Design review of the part built by this model. Coordinates are the model's own, in mm. Face numbers are marked on the shaded views. A direction names the side the tool comes from. Coordinates: 2 decimals unless noted, no trailing zeros. Loops run counter-clockwise (first coordinate to the right, second up) from the corner with the lowest first, then second, coordinate; pieces in that order, holes last. Notation, with made-up numbers: (45, -0.5) -> (87, -0.5) arc R15 cw to (87, 5.5) -> close; hole circle Ø3 at (-14.5, -9). An arc over 180 degrees is marked (long way). Use one line per item in the form item = value. Start each with the question number.
1. Consider section D-D (x = 3.5). State the section outline as (y, z) points, then the cut area to 3 significant figures.
2. Wall thickness on line 1 (Y direction, x = -13.65, z = 73.05) (3 decimals); line 2 (Y direction, x = 19.4, z = 25.05); line 3 (Z direction, x = -13, y = -13): over which ranges is each line inside the solid? List them lowest first. Write a range as from..to.
3. Machinability: for the marked faces 1, 2 and 3, which of the approach directions +Z, -Z, +X, -X, +Y, -Y give a long, thin tool a straight path to every point of the face, cutting with its end or side? Answer none if there is none.
4. Consider section B-B (y = 29.95). State the section outline as (x, z) points (3 decimals).
5. Consider section A-A (x = 17.47). State the section outline as (y, z) points.
6. Consider section C-C (z = 53). State the section outline as (x, y) points (3 decimals).
7. For pin 1 (2 mm diameter, centred on y = 4, z = 44.5, fed in from -X); pin 2 (12 mm diameter, centred on x = 10, z = 56, fed in from +Y); pin 3 (1.6 mm diameter, centred on x = 12.5, y = 6, fed in from +Z); pin 4 (2 mm diameter, centred on y = 29.95, z = 73.05, fed in from -X), all flat-tipped, find the tip position at first contact; note any pin that passes through.
from build123d import *

# Parameters (mm, degrees)
SKETCH1_W           = 11
SKETCH1_H           = 17
SKETCH1_W_2         = 7
SKETCH1_H_2         = 13
BOSS_EXTRUDE1_DEPTH = 76.2
SKETCH2_W           = 11
SKETCH2_H           = 17
BOSS_EXTRUDE2_DEPTH = 2
SKETCH3_W           = 7
SKETCH3_H           = 11
CUT_EXTRUDE1_DEPTH  = 2
SKETCH4_W           = 38.1
SKETCH4_H           = 38.1
SKETCH4_W_2         = 11
SKETCH4_H_2         = 17
BOSS_EXTRUDE3_DEPTH = 3
SKETCH5_R           = 12.7
SKETCH5_W           = 11
SKETCH5_H           = 17
BOSS_EXTRUDE4_DEPTH = 2.54
SKETCH6_W           = 11
SKETCH6_H           = 58.214
BOSS_EXTRUDE5_DEPTH = 6.35
CUT_EXTRUDE2_REACH  = 87.303
SKETCH7_R           = 3.302
SKETCH8_W           = 6.985
SKETCH8_H           = 31.75
CUT_EXTRUDE3_DEPTH  = 6.35
SKETCH9_W           = 58.42
SKETCH9_H           = 12.7
BOSS_EXTRUDE6_DEPTH = 12.7
SKETCH10_W          = 3.175
SKETCH10_H          = 58.214
BOSS_EXTRUDE7_DEPTH = 20
SKETCH11_R          = 1.778
SKETCH11_W          = 3.884096392
SKETCH11_H          = 20
CUT_EXTRUDE4_DEPTH  = 91.512682122
FILLET1_R           = 1.27
CHAMFER1_SIZE       = 11.43
FILLET3_R           = 2.54
SKETCH12_W          = 58.214
SKETCH12_H          = 11.675
BOSS_EXTRUDE8_DEPTH = 12.7
SKETCH13_W          = 3.175
SKETCH13_H          = 54.356
BOSS_EXTRUDE9_DEPTH = 20
CHAMFER3_SIZE       = 12.7
FILLET4_R           = 2.54
SKETCH14_W          = 6.096
SKETCH14_H          = 28.594092226
CUT_EXTRUDE5_DEPTH  = 6.35
SKETCH15_R          = 1.778
CUT_EXTRUDE6_DEPTH  = 91.512682122
FILLET5_R           = 1.27
SKETCH16_R          = 1.5875
CUT_EXTRUDE7_DEPTH  = 12.7
FILLET6_R           = 2.54
SKETCH17_R          = 3.302
CUT_EXTRUDE8_DEPTH  = 72.570750283
SKETCH19_W          = 11
SKETCH19_H          = 17
CUT_EXTRUDE9_DEPTH  = 2.032
SKETCH21_W          = 41.629903608
SKETCH21_H          = 20
CUT_EXTRUDE10_DEPTH = 25.4
SKETCH22_W          = 41.656
SKETCH22_H          = 20
CUT_EXTRUDE11_DEPTH = 25.4


with BuildPart() as part:
    # Sketch1 → Boss-Extrude1 (new body)
    with BuildSketch(Plane.XY):
        with Locations((3.5, 6.5)):
            Rectangle(SKETCH1_W, SKETCH1_H)
        with Locations((3.5, 6.5)):
            Rectangle(SKETCH1_W_2, SKETCH1_H_2, mode=Mode.SUBTRACT)
    extrude(amount=BOSS_EXTRUDE1_DEPTH)

    # Sketch2 → Boss-Extrude2 (add)
    with BuildSketch(Plane(origin=(0, 0, 0), x_dir=(-1, 0, 0), z_dir=(0, 0, -1))):
        with Locations((-3.5, 6.5)):
            Rectangle(SKETCH2_W, SKETCH2_H)
    extrude(amount=BOSS_EXTRUDE2_DEPTH)

    # Sketch3 → Cut-Extrude1 (cut)
    with BuildSketch(Plane(origin=(0, -2, 0), x_dir=(-1, 0, 0), z_dir=(0, -1, 0))):
        with Locations((-3.5, -5.5)):
            Rectangle(SKETCH3_W, SKETCH3_H)
    extrude(amount=-CUT_EXTRUDE1_DEPTH, mode=Mode.SUBTRACT)

    # Sketch4 → Boss-Extrude3 (add)
    with BuildSketch(Plane.XY.offset(14.986)):
        with Locations((3.5, 6.5)):
            Rectangle(SKETCH4_W, SKETCH4_H)
        with Locations((3.5, 6.5)):
            Rectangle(SKETCH4_W_2, SKETCH4_H_2, mode=Mode.SUBTRACT)
    extrude(amount=BOSS_EXTRUDE3_DEPTH)

    # Sketch5 → Boss-Extrude4 (add)
    with BuildSketch(Plane(origin=(0, 0, 14.986), x_dir=(-1, 0, 0), z_dir=(0, 0, -1))):
        with Locations(Location((-3.5, 6.5, 0), (0, 0, 180))):
            Circle(SKETCH5_R)
        with Locations((-3.5, 6.5)):
            Rectangle(SKETCH5_W, SKETCH5_H, mode=Mode.SUBTRACT)
    extrude(amount=BOSS_EXTRUDE4_DEPTH)

    # Sketch6 → Boss-Extrude5 (add)
    with BuildSketch(Plane.XZ.offset(2)):
        with Locations((3.5, 47.093)):
            Rectangle(SKETCH6_W, SKETCH6_H)
    extrude(amount=BOSS_EXTRUDE5_DEPTH)

    # Cut-Extrude2: up to this face of the body (flat: up to its plane)
    cut_extrude2_end = Plane(part.part.faces().sort_by_distance((3.5, 6.5, -2))[0])
    # Sketch7 → Cut-Extrude2 (cut, up to the picked face)
    with BuildSketch(Plane.XY.offset(76.2), mode=Mode.PRIVATE) as cut_extrude2_sk1:
        with Locations((3.461, -3.429)):
            Circle(SKETCH7_R)
    cut_extrude2_tool1 = split(extrude(cut_extrude2_sk1.sketch, amount=-CUT_EXTRUDE2_REACH, mode=Mode.PRIVATE), bisect_by=cut_extrude2_end, keep=Keep.BOTH, mode=Mode.PRIVATE)
    add(cut_extrude2_tool1.solids().sort_by(Axis((3.461, -3.429, 76.2), (0, 0, -1)))[0], mode=Mode.SUBTRACT)

    # Sketch8 → Cut-Extrude3 (cut)
    with BuildSketch(Plane(origin=(0, 15, 0), x_dir=(1, 0, 0), z_dir=(0, 1, 0))):
        with Locations((3.4925, -60.325)):
            Rectangle(SKETCH8_W, SKETCH8_H)
    extrude(amount=-CUT_EXTRUDE3_DEPTH, mode=Mode.SUBTRACT)

    # Sketch9 → Boss-Extrude6 (add)
    with BuildSketch(Plane(origin=(9, 0, 0), x_dir=(0, 0, -1), z_dir=(1, 0, 0))):
        with Locations((-46.99, 8.65)):
            Rectangle(SKETCH9_W, SKETCH9_H)
    extrude(amount=BOSS_EXTRUDE6_DEPTH)

    # Sketch10 → Boss-Extrude7 (add)
    with BuildSketch(Plane(origin=(0, 15, 0), x_dir=(1, 0, 0), z_dir=(0, 1, 0))):
        with Locations((20.1125, -47.093)):
            Rectangle(SKETCH10_W, SKETCH10_H)
    extrude(amount=BOSS_EXTRUDE7_DEPTH)

    # Sketch11 → Cut-Extrude4 (cut, through all)
    with BuildSketch(Plane.ZY.offset(-18.525)):
        with Locations((25.05, 29.95)):
            Circle(SKETCH11_R)
        with Locations((25.05, 20.05)):
            Circle(SKETCH11_R)
        with Locations((73.05, 29.95)):
            Circle(SKETCH11_R)
        with Locations((73.05, 20.05)):
            Circle(SKETCH11_R)
        with Locations((19.928048196, 25)):
            Rectangle(SKETCH11_W, SKETCH11_H)
    extrude(amount=-CUT_EXTRUDE4_DEPTH, mode=Mode.SUBTRACT)

    # Fillet1
    fillet1_edges = [part.edges().sort_by_distance(p)[0] for p in [
        (20.1125, 35, 76.2),
        (20.1125, 35, 21.870096392),
    ]]
    fillet(fillet1_edges, radius=FILLET1_R)

    # Chamfer1
    # the kernel refuses this chamfer: 11.43 mm, written as the material it adds along each edge
    with BuildSketch(Plane(origin=(9, 2.3, 17.986), x_dir=(0.9996219169112968, 0.027495876610586382, 0), z_dir=(0, 0, 1))) as chamfer1_piece_1_section:
        Polygon((CHAMFER1_SIZE * 0.999621916911, -CHAMFER1_SIZE * 0.0274958766106), (-CHAMFER1_SIZE * 0.0274958766106, -CHAMFER1_SIZE * 0.999621916911), (0, 0), align=None)
    chamfer1_piece_1 = extrude(amount=58.214, mode=Mode.PRIVATE)
    chamfer1_piece_1 = split(chamfer1_piece_1, bisect_by=Plane(origin=(13.789958752, -8.35, 47.093), z_dir=(0, 1, 0)), keep=Keep.TOP, mode=Mode.PRIVATE)
    add(chamfer1_piece_1)

    # Fillet3
    fillet3_edges = [part.edges().sort_by_distance(p)[0] for p in [
        (20.43, 2.3, 47.093),
        (9.78, -8.35, 47.093),
    ]]
    fillet(fillet3_edges, radius=FILLET3_R)

    # Sketch12 → Boss-Extrude8 (add)
    with BuildSketch(Plane.ZY.offset(2)):
        with Locations((47.093, -2.5125)):
            Rectangle(SKETCH12_W, SKETCH12_H)
    extrude(amount=BOSS_EXTRUDE8_DEPTH)

    # Sketch13 → Boss-Extrude9 (add)
    with BuildSketch(Plane.XZ.offset(8.35)):
        with Locations((-13.1125, 49.022)):
            Rectangle(SKETCH13_W, SKETCH13_H)
    extrude(amount=BOSS_EXTRUDE9_DEPTH)

    # Chamfer3
    # the kernel refuses this chamfer: 12.7 mm, written as the material it adds along each edge
    with BuildSketch(Plane(origin=(-2, 3.325, 17.986), x_dir=(0.027495876610586365, 0.9996219169112966, 0), z_dir=(0, 0, 1))) as chamfer3_piece_1_section:
        Polygon((CHAMFER3_SIZE * 0.999621916911, CHAMFER3_SIZE * 0.0274958766106), (-CHAMFER3_SIZE * 0.0274958766106, CHAMFER3_SIZE * 0.999621916911), (0, 0), align=None)
    chamfer3_piece_1 = extrude(amount=58.214, mode=Mode.PRIVATE)
    chamfer3_piece_1 = split(chamfer3_piece_1, bisect_by=Plane(origin=(-6.232956887, 15, 47.093), z_dir=(0, -1, 0)), keep=Keep.TOP, mode=Mode.PRIVATE)
    chamfer3_piece_1 = split(chamfer3_piece_1, bisect_by=Plane(origin=(-14.7, 7.408033371, 47.093), z_dir=(1, 0, 0)), keep=Keep.TOP, mode=Mode.PRIVATE)
    add(chamfer3_piece_1)

    # Fillet4
    fillet4_edges = [part.edges().sort_by_distance(p)[0] for p in [
        (-14.7, 3.325, 47.093),
        (-3.025, 15, 47.093),
    ]]
    fillet(fillet4_edges, radius=FILLET4_R)

    # Sketch14 → Cut-Extrude5 (cut)
    with BuildSketch(Plane.XZ.offset(8.35)):
        with Locations((3.647897552, 55.896932406)):
            Rectangle(SKETCH14_W, SKETCH14_H)
    extrude(amount=-CUT_EXTRUDE5_DEPTH, mode=Mode.SUBTRACT)

    # Sketch15 → Cut-Extrude6 (cut, through all)
    with BuildSketch(Plane(origin=(-11.525, 0, 0), x_dir=(0, 0, -1), z_dir=(1, 0, 0))):
        with Locations((-73.05, -13.4)):
            Circle(SKETCH15_R)
        with Locations((-73.05, -23.3)):
            Circle(SKETCH15_R)
        with Locations((-25.05, -13.4)):
            Circle(SKETCH15_R)
        with Locations((-25.05, -23.3)):
            Circle(SKETCH15_R)
    extrude(amount=-CUT_EXTRUDE6_DEPTH, mode=Mode.SUBTRACT)

    # Fillet5
    fillet5_edges = [part.edges().sort_by_distance(p)[0] for p in [
        (-13.1125, -28.35, 21.844),
        (-13.1125, -28.35, 76.2),
    ]]
    fillet(fillet5_edges, radius=FILLET5_R)

    # Sketch16 → Cut-Extrude7 (cut)
    with BuildSketch(Plane.XY.offset(76.2)):
        with Locations((-6.016625, 5.971505071)):
            Circle(SKETCH16_R)
        with Locations((13.033375, 5.971505071)):
            Circle(SKETCH16_R)
    extrude(amount=-CUT_EXTRUDE7_DEPTH, mode=Mode.SUBTRACT)

    # Fillet6
    fillet6_edges = [part.edges().sort_by_distance(p)[0] for p in [
        (-15.55, 25.55, 16.486),
        (-15.55, -12.55, 16.486),
        (22.55, -12.55, 16.486),
        (22.55, 25.55, 16.486),
    ]]
    fillet(fillet6_edges, radius=FILLET6_R)

    # Sketch17 → Cut-Extrude8 (cut, through all)
    with BuildSketch(Plane.XY.offset(17.986)):
        with Locations((-10.47, 20.47)):
            Circle(SKETCH17_R)
        with Locations((17.47, -7.47)):
            Circle(SKETCH17_R)
    extrude(amount=-CUT_EXTRUDE8_DEPTH, mode=Mode.SUBTRACT)

    # Sketch19 → Cut-Extrude9 (cut)
    with BuildSketch(Plane(origin=(0, 0, -2), x_dir=(-1, 0, 0), z_dir=(0, 0, -1))):
        with Locations((-3.5, 6.5)):
            Rectangle(SKETCH19_W, SKETCH19_H)
    extrude(amount=-CUT_EXTRUDE9_DEPTH, mode=Mode.SUBTRACT)

    # Sketch21 → Cut-Extrude10 (cut)
    with BuildSketch(Plane(origin=(21.7, 0, 0), x_dir=(0, 0, -1), z_dir=(1, 0, 0))):
        with Locations((-49.035048196, 25)):
            Rectangle(SKETCH21_W, SKETCH21_H)
    extrude(amount=-CUT_EXTRUDE10_DEPTH, mode=Mode.SUBTRACT)

    # Sketch22 → Cut-Extrude11 (cut)
    with BuildSketch(Plane.ZY.offset(14.7)):
        with Locations((49.022, -18.35)):
            Rectangle(SKETCH22_W, SKETCH22_H)
    extrude(amount=-CUT_EXTRUDE11_DEPTH, mode=Mode.SUBTRACT)


solid = part.part
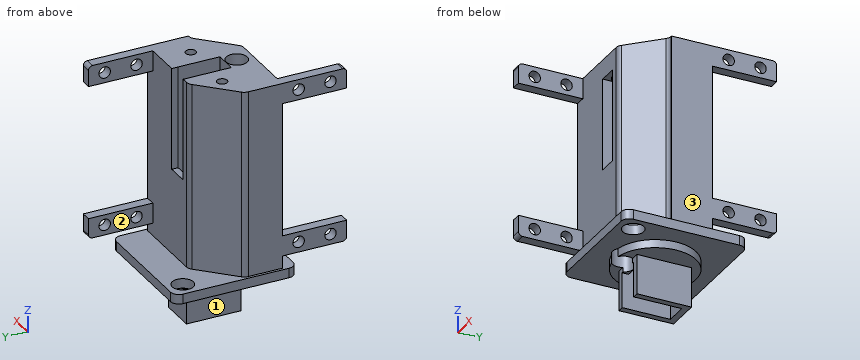
Geometry check:
q1.outline = (-12.55, 14.99) -> (-6.73, 14.99) -> (-6.73, 41.6) -> (-8.35, 41.6) -> (-8.35, 17.99) -> (-12.55, 17.99) -> close; (-8.35, 70.19) -> (-6.73, 70.19) -> (-6.73, 76.2) -> (-8.35, 76.2) -> close; (-0.13, 11) -> (0, 11) -> (0, 76.2) -> (-0.13, 76.2) -> close; (13, 0.03) -> (15, 0.03) -> (15, 12.45) -> (19.2, 12.45) -> (19.2, 14.99) -> (25.55, 14.99) -> (25.55, 17.99) -> (15, 17.99) -> (15, 44.45) -> (13, 44.45) -> close
q1.area = 205 mm²
q2.line_1 = -28.35..-25.078, -21.522..-15.178, -11.622..4.375
q2.line_2 = 1.27..18.27, 21.83..28.17, 31.73..35
q2.line_3 = 21.84..23.32, 26.78..28.19, 69.85..71.32, 74.78..76.2
q3.face_1 = -Z, -X, +Y, -Y
q3.face_2 = +Z, -X, +Y
q3.face_3 = +Z, +X, +Y, -Y
q4.outline = (18.525, 21.87) -> (21.7, 21.87) -> (21.7, 23.272) -> (18.525, 23.272) -> close; (18.525, 26.828) -> (21.7, 26.828) -> (21.7, 28.22) -> (18.525, 28.22) -> close; (18.525, 69.85) -> (21.7, 69.85) -> (21.7, 71.272) -> (18.525, 71.272) -> close; (18.525, 74.828) -> (21.7, 74.828) -> (21.7, 76.2) -> (18.525, 76.2) -> close
q5.outline = (-12.55, 14.99) -> (-10.77, 14.99) -> (-10.77, 17.99) -> (-12.55, 17.99) -> close; (-4.17, 14.99) -> (25.55, 14.99) -> (25.55, 17.99) -> (15, 17.99) -> (15, 76.2) -> (-0.66, 76.2) -> (-0.66, 17.99) -> (-4.17, 17.99) -> close
q6.outline = (-14.7, -8.35) -> (0.6, -8.35) -> (0.6, -5.077) arc R3.302 cw (long way) to (6.438, -2) -> (6.696, -2) -> (6.696, -2.767) arc R3.302 cw to (6.696, -4.091) -> (6.696, -8.35) -> (8.728, -8.35) arc R2.54 ccw to (10.524, -7.606) -> (19.686, 1.556) arc R2.54 cw to (21.482, 2.3) -> (21.7, 2.3) -> (21.7, 15) -> (6.985, 15) -> (6.985, 13) -> (7, 13) -> (7, 0) -> (0, 0) -> (0, 15) -> (-1.973, 15) arc R2.54 ccw to (-3.769, 14.256) -> (-13.956, 4.069) arc R2.54 ccw to (-14.7, 2.273) -> close
q7.pin_1 = -14.59
q7.pin_2 = 15
q7.pin_3 = 63.5
q7.pin_4 = through
